Could you check a few things on this drawing? It's one solid part, dimensions in mm from its lowest x, y, z. A direction names the side the tool comes from. Give positions to 0.01 mm unless a question says otherwise; leave off trailing zeros. Loops run counter-clockwise (first coordinate to the right, second up) from the corner with the lowest first, then second, coordinate; pieces in that order, holes last. Notation, with made-up numbers: (52.5, 21.25) - (77.5, 21.25) arc R21 ccw to (77.5, 59.25) - close; hole circle Ø11 at (22, 86.5). An arc over 180 degrees is marked (long way). Answer as a JSON object with one key per item and string values.
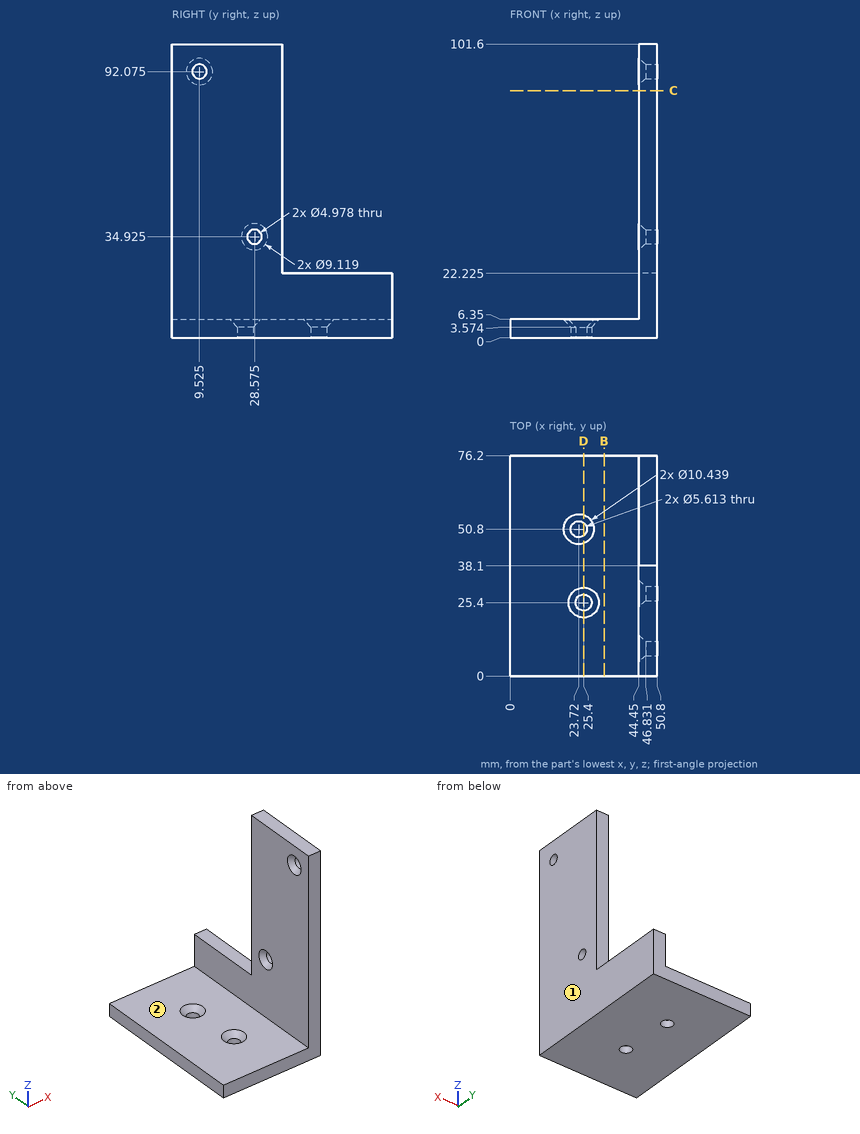
1) I need wall thicknesses on L1, parallel to X at y = 50.8, z = 0.9; L2, parallel to X at y = 67.5, z = 7.5; L3, parallel to Z at x = 42, y = 25.5. Which ranges of each line are inside material? Lowest first, please.
Check sheet entries:
{"L1": "0 to 20.91, 26.53 to 50.8", "L2": "44.45 to 50.8", "L3": "0 to 6.35"}
2) Imagine slicing it at B-B on x = 32.5. Write out the boundary of the cut face in (y, z).
Check sheet entries:
{"outline": "(0, 0) - (76.2, 0) - (76.2, 6.35) - (0, 6.35) - close"}
3) Imagine slicing it at C-C on z = 85.5. Write out the boundary of the cut face in (x, y), and give its area (3 significant figures).
Check sheet entries:
{"outline": "(44.45, 0) - (50.8, 0) - (50.8, 38.1) - (44.45, 38.1) - close", "area": "242 mm2"}
4) I'm going to push flat-ended pins straight in: P1, Ø5, axis at x = 47.5, z = 47.5, coming from the +Y side; P2, Ø5, axis at x = 43.5, z = 29.5, coming from the -Y side; P3, Ø8, axis at y = 28.575, z = 34.925, coming from the -X side (1 decimal); P4, Ø1, axis at y = 32, z = 12, coming from the -X side. Where does each tip first touch, or does it pass through?
Check sheet entries:
{"P1": "y = 38.1", "P2": "y = 0", "P3": "x = 45.1", "P4": "x = 44.45"}
5) Which directions (+Z, -Z, +X, -X, +Y, -Y) give clear straight access to the entire face, cutting with the end or side of a thin tool? Please do the marked faces 1 and 2.
Check sheet entries:
{"face 1": "+Z, -Z, +X, +Y, -Y", "face 2": "+Z, -X, +Y, -Y"}
6) Imagine slicing it at D-D on x = 25.4. Give the number of separate pieces and of enclosed holes in the cut face, and give its area (3 significant figures).
Check sheet entries:
{"separate pieces": "3", "enclosed holes": "0", "area": "405 mm2"}
